from build123d import *

# Parameters (mm, degrees)
SKETCH002_R    = 4.6
PAD_DEPTH      = 5
PAD_DEPTH_BACK = 5


with BuildPart() as pad:
    # Sketch002 → Pad (new body, two sides)
    with BuildSketch(Plane.XZ) as pad_sk:
        with BuildLine():
            Line((-30, 0), (-47, 0))
            ThreePointArc((-47, 0), (-54.870528, -8.731056), (-49, -18.915037))
            Line((-49, -18.915037), (-36, -22))
            Line((-36, -22), (-30, 0))
        make_face()
        with Locations((-44.925964, -9.782555)):
            Circle(SKETCH002_R, mode=Mode.SUBTRACT)
    extrude(amount=PAD_DEPTH)
    extrude(pad_sk.sketch, amount=-PAD_DEPTH_BACK)


with BuildPart() as fusion:
    # Sketch001 → Revolution (revolve)
    with BuildSketch(Plane.XZ):
        Polygon((-20.5, 0), (-33, 0), (-39.4, -30), (-43.062567, -51.544511), (-46.2, -70), (-48, -90), (-50, -135), (-49, -135), (-47, -90), (-45, -70), (-38, -30), (-30, -5), (-20.5, -5), align=None)
    revolve(axis=Axis((0, 0, 0), (0, 0, 1)))

    # Fusion: union Pad
    add(pad.part)


solid = fusion.part
Can you work these out from the model? Positions are in its coordinate system, mm. A direction names the side the tool comes from. Round coordinates to 2 decimals unless told otherwise and drop trailing zeros. Loops run counter-clockwise (first coordinate to the right, second up) from the corner with the lowest first, then second, coordinate; pieces in that order, holes last. Notation, with made-up numbers: (-19, 69.25) - (2, 69.25) arc R30 ccw to (2, 91.25) - close; hole circle Ø1 at (20, -20.5). An arc over 180 degrees is marked (long way). Use CSV: the item, a comma, the result in double quotes. Start each with the question number.
1) We'd pull the mould along Y, two halves only. Please class faces 1 (the cylindrical face through (4.444, 20.013, -2.465)), 2 (the flat face through (-41, 5, -13)), 3 (the conical face through (7.549, 33.995, -8.543)): released by +Y, released by -Y, zero draft, split by the parting line, or undercut.
2) If we section it at A-A on z = -74: Write out the boundary of the cut face in (x, y), plus the area to 3 significant figures.
3) For faces 4 (the flat face through (-20, 6, -5)), 5 (the cylindrical face through (-40.54, 0.07, -8.4)), 6 (the flat face through (-41, -5, -13)), which set-ups out of +Z, -Z, +X, -X, +Y, -Y let a thin tool reach every point of the face, with its end or its side?
4) Please list where these lines run through material, in increasing order: probe 1 along X at (y, z) = (-1.5, -79); probe 2 along Y at (x, z) = (10, -47); probe 3 along X at (y, z) = (16, -42). Write a range as [from, to].
5) For pin 1 Ø4 at (y, z) = (4.5, -72) entering from -X; pin 2 Ø12 at (x, z) = (-21, -79) entering from -Y; pin 3 Ø12 at (y, z) = (23, -89.5) entering from -X; pin 4 Ø6.5 at (x, z) = (-44, -10.5) entering from -Y, each with a flat end and sliding along its axis, tell me the tip position at first contact or that it passes through.
6) If we section it at B-B on z = -27: Write out the boundary of the cut face in (x, y), plus the area to 3 significant figures.
Geometry results:
1,face 1,"undercut"
1,face 2,"released by +Y"
1,face 3,"split by the parting line"
2,outline,"circle Ø93.12 at (0, 0); hole circle Ø90.8 at (0, 0)"
2,area,"335 mm2"
3,face 4,"-Z"
3,face 5,"+Y, -Y"
3,face 6,"+Z, -X, -Y"
4,probe 1,"x = [-46.99, -45.88], [45.88, 46.99]"
4,probe 2,"y = [-41.09, -39.74], [39.74, 41.09]"
4,probe 3,"x = [-38.23, -36.77], [36.77, 38.23]"
5,pin 1,"stops at x = -46.41"
5,pin 2,"stops at y = -44.63"
5,pin 3,"stops at x = -44.88"
5,pin 4,"passes through"
6,outline,"circle Ø77.52 at (0, 0); hole circle Ø74.08 at (0, 0)"
6,area,"410 mm2"
